Can you work these out from the model? Positions are in its coordinate system, mm. Face numbers are marked on the shaded views. A direction names the side the tool comes from. Round coordinates to 2 decimals unless told otherwise and drop trailing zeros. Order: outer loops, then holes, each group sorted by start corner. A loop starts at its lowest first (then second) coordinate and runs counter-clockwise, first axis right, second up. Notation, with made-up numbers: (-5, 78) -> (36, 78) arc R21 ccw to (36, 82) -> close; hole circle Ø3 at (57.25, 26.5). An arc over 180 degrees is marked (long way). One line per item, written item: value.
```python
from build123d import *

# Parameters (mm, degrees)
SKETCH1_W           = 15
SKETCH1_H           = 15
BOSS_EXTRUDE1_DEPTH = 15
BOSS_EXTRUDE2_START = -7.5
SKETCH3_R           = 5
BOSS_EXTRUDE2_DEPTH = 50
BOSS_EXTRUDE3_START = -7.5
SKETCH4_R           = 5
BOSS_EXTRUDE3_DEPTH = 50
CHAMFER1_SIZE       = 0.5


with BuildPart() as part:
    # Sketch1 → Boss-Extrude1 (new body)
    with BuildSketch(Plane.XY):
        Rectangle(SKETCH1_W, SKETCH1_H)
    extrude(amount=BOSS_EXTRUDE1_DEPTH)

    # Sketch3 → Boss-Extrude2 (add, symmetric)
    with BuildSketch(Plane(origin=(7.5, 0, 0), x_dir=(0, 0, -1), z_dir=(1, 0, 0)).offset(BOSS_EXTRUDE2_START)):
        with Locations(Location((-7.5, 0, 0), (0, 0, 90))):
            Circle(SKETCH3_R)
    extrude(amount=BOSS_EXTRUDE2_DEPTH, both=True)

    # Sketch4 → Boss-Extrude3 (add, symmetric)
    with BuildSketch(Plane.XY.offset(15).offset(BOSS_EXTRUDE3_START)):
        Circle(SKETCH4_R)
    extrude(amount=BOSS_EXTRUDE3_DEPTH, both=True)

    # Chamfer1
    chamfer1_edges = [part.edges().sort_by_distance(p)[0] for p in [
        (-7.5, 0, 15),
        (-50, -5, 7.5),
        (50, -5, 7.5),
        (0, -7.5, 15),
        (-5, 0, -42.5),
        (-5, 0, 57.5),
        (7.5, 0, 15),
        (0, -7.5, 0),
        (-7.5, 0, 0),
        (7.5, 0, 0),
        (7.5, -7.5, 7.5),
        (-7.5, -7.5, 7.5),
        (-7.5, 7.5, 7.5),
        (7.5, 7.5, 7.5),
        (0, 7.5, 15),
    ]]
    chamfer(chamfer1_edges, length=CHAMFER1_SIZE)


solid = part.part
```
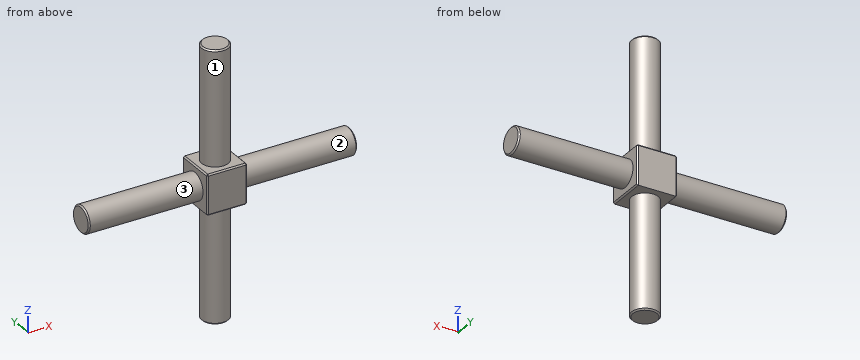
Q1. I want a section at D-D on z = -15. List the corners of the cut face in (x, y) for me, plus the area to 3 significant figures.
Answers below:
outline: circle Ø10 at (0, 0)
area: 78.5 mm^2
Q2. Will these pins go through, and if not, where does the flat tip stop? pin 1 Ø4 at (y, z) = (3.5, -23) entering from +X; pin 2 Ø1.5 at (y, z) = (3.5, 11.5) entering from -X; pin 3 Ø1.5 at (x, y) = (20, 1.5) entering from +Z.
Answers below:
pin 1: x = 4.77
pin 2: x = -49.93
pin 3: z = 12.44
Q3. I want a section at A-A on z = 7.5. List the corners of the cut face in (x, y) for me.
Answers below:
outline: (-50, -4.5) -> (-49.5, -5) -> (-7.5, -5) -> (-7.5, -7) -> (-7, -7.5) -> (7, -7.5) -> (7.5, -7) -> (7.5, -5) -> (49.5, -5) -> (50, -4.5) -> (50, 4.5) -> (49.5, 5) -> (7.5, 5) -> (7.5, 7) -> (7, 7.5) -> (-7, 7.5) -> (-7.5, 7) -> (-7.5, 5) -> (-49.5, 5) -> (-50, 4.5) -> close
Q4. Please list where these lines run through material, in increasing order: line 1 along Z through (x, y) = (4, 6.5); line 2 along X through (y, z) = (-3, -20.5); line 3 along X through (y, z) = (4, -27).
Answers below:
line 1: 0 to 15
line 2: -4 to 4
line 3: -3 to 3
Q5. I want a section at B-B on x = 0. List the corners of the cut face in (y, z) for me.
Answers below:
outline: (-7.5, 0.5) -> (-7, 0) -> (-5, 0) -> (-5, -42) -> (-4.5, -42.5) -> (4.5, -42.5) -> (5, -42) -> (5, 0) -> (7.5, 0) -> (7.5, 14.5) -> (7, 15) -> (5, 15) -> (5, 57) -> (4.5, 57.5) -> (-4.5, 57.5) -> (-5, 57) -> (-5, 15) -> (-7, 15) -> (-7.5, 14.5) -> close
Q6. On a 3-axis mill with a long thin cutter (end or side, diameter ignored), from which of +Z, -Z, +X, -X, +Y, -Y can I reach the whole of each face in a straight line? I mean the marked faces 1, 2 and 3. Say none if no direction works.
Answers below:
face 1: +Z
face 2: +X
face 3: -X
